The listing builds one solid part. Answer for the finished solid, in the listing's coordinates (mm). Face numbers are marked on the shaded views. Coordinates: 2 decimals unless noted, no trailing zeros. Order: outer loops, then holes, each group sorted by start corner. A loop starts at its lowest first (then second) coordinate and runs counter-clockwise, first axis right, second up. Notation, with made-up numbers: (16.25, -37) - (59.25, -37) arc R13 ccw to (59.25, -27) - close; hole circle Ø4 at (88, 51.5). An arc over 180 degrees is marked (long way). One line per item, written item: value. Start each with the question number.
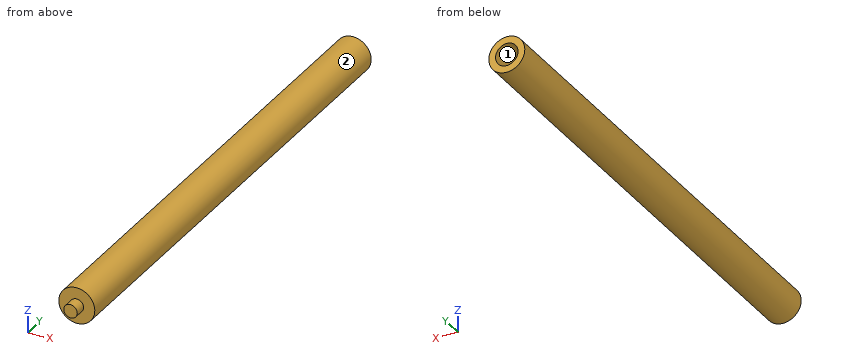
```python
from build123d import *

# Parameters (mm, degrees)
SKETCH1_R           = 4
BOSS_EXTRUDE1_DEPTH = 40
SKETCH2_R           = 1.5
BOSS_EXTRUDE2_DEPTH = 2.5
BOSS_EXTRUDE3_START = 70
SKETCH3_R           = 4
BOSS_EXTRUDE3_DEPTH = 70
SKETCH4_R           = 2.5
CUT_EXTRUDE1_DEPTH  = 10


with BuildPart() as part:
    # Sketch1 → Boss-Extrude1 (new body)
    with BuildSketch(Plane(origin=(0, 0, 0), x_dir=(1, 0, 0), z_dir=(0, 1, 0))):
        with Locations(Location((0, 0, 0), (0, 0, 270))):
            Circle(SKETCH1_R)
    extrude(amount=-BOSS_EXTRUDE1_DEPTH)

    # Sketch2 → Boss-Extrude2 (add)
    with BuildSketch(Plane.XZ.offset(40)):
        with Locations(Location((0, 0, 0), (0, 0, 270))):
            Circle(SKETCH2_R)
    extrude(amount=BOSS_EXTRUDE2_DEPTH)

    # Sketch3 → Boss-Extrude3 (add)
    with BuildSketch(Plane(origin=(0, 0, 0), x_dir=(1, 0, 0), z_dir=(0, 1, 0)).offset(BOSS_EXTRUDE3_START)):
        with Locations(Location((0, 0, 0), (0, 0, 270))):
            Circle(SKETCH3_R)
    extrude(amount=-BOSS_EXTRUDE3_DEPTH)

    # Sketch4 → Cut-Extrude1 (cut)
    with BuildSketch(Plane(origin=(0, 70, 0), x_dir=(1, 0, 0), z_dir=(0, 1, 0))):
        with Locations(Location((0, 0, 0), (0, 0, 270))):
            Circle(SKETCH4_R)
    extrude(amount=-CUT_EXTRUDE1_DEPTH, mode=Mode.SUBTRACT)


solid = part.part
```
(1) The part is cut by section A-A on x = 0. Determine the outline of the cut face in (y, z), plus the area to 4 significant figures.
(2) The part is cut by section B-B on z = 0. Determine the outline of the cut face in (x, y), plus the area to 4 significant figures.
(3) Consider probe 1 along X at (y, z) = (63.75, 0); probe 2 along Y at (x, z) = (-1.5, 1.5); probe 3 along Y at (x, z) = (-3, 0.5). Determine where each line is inside the solid, lowest interval first.
(4) Flat-ended cylindrical pins translate along their axes: pin 1 Ø1.5 at (x, z) = (0.5, 0) entering from +Y; pin 2 Ø3 at (x, y) = (-2.5, 16) entering from -Z. Find the tip coordinate at first contact, or state that the pin passes through.
(5) For a pull along Z with two mould halves and no side action, classify the marked faces 1 and 2 as pulls with the +Z half, pulls with the -Z half, needs draft (parallel to the pull), parting line crosses it, or undercut.
(6) The part is cut by section C-C on y = -21.5. Determine the outline of the cut face in (x, z).
Completed:
1. outline: (-42.5, -1.5) - (-40, -1.5) - (-40, -4) - (70, -4) - (70, -2.5) - (60, -2.5) - (60, 2.5) - (70, 2.5) - (70, 4) - (-40, 4) - (-40, 1.5) - (-42.5, 1.5) - close
1. area: 837.5 mm2
2. outline: (-4, -40) - (-1.5, -40) - (-1.5, -42.5) - (1.5, -42.5) - (1.5, -40) - (4, -40) - (4, 70) - (2.5, 70) - (2.5, 60) - (-2.5, 60) - (-2.5, 70) - (-4, 70) - close
2. area: 837.5 mm2
3. probe 1: x = -4 to -2.5, 2.5 to 4
3. probe 2: y = -40 to 60
3. probe 3: y = -40 to 70
4. pin 1: stops at y = 60
4. pin 2: stops at z = -3.87
5. face 1: undercut
5. face 2: parting line crosses it
6. outline: circle Ø8 at (0, 0)
